Build history of the part. All positions in model axes, mm. A direction names the side the tool comes from. Round coordinates to 2 decimals unless told otherwise and drop trailing zeros. Write each loop counter-clockwise with the first axis right and the second up, starting at its lowest first coordinate (ties: lowest second). Pieces come first, ordered by that corner, then holes. Notation, with made-up numbers: M 57.5,-31 L 108.5,-31 A25 cw 108.5,-12 Z; hole C 39.25,-27.75 d2. An arc over 180 degrees is marked long. Use a Markdown table: item, result.
from build123d import *

# Parameters (mm, degrees)
FLOOR_2_DEPTH        = 40
SIDE_START           = 37
SKETCH_2_W           = 197.5
SKETCH_2_H           = 35
SIDE_FRONT_DEPTH     = 3
SIDE_START_2         = -37
SKETCH_3_W           = 197.5
SKETCH_3_H           = 35
SIDE_REAR_DEPTH      = 3
INSIDE_BEND_FRONT_R  = 3
INSIDE_BEND_REAR_R   = 3
OUTSIDE_BEND_FRONT_R = 6
OUTSIDE_BEND_REAR_R  = 6
JOINT_START          = 40
SKETCH_4_W           = 45
SKETCH_4_H           = 21
JOINT_FRONT_DEPTH    = 3
JOINT_START_2        = -40
SKETCH_5_W           = 45
SKETCH_5_H           = 21
JOINT_REAR_DEPTH     = 3
SKETCH_6_R           = 2.5
FIXING_HOLES_DEPTH   = 43


with BuildPart() as part:
    # 草图1 → Floor 2 (new, symmetric)
    with BuildSketch(Plane.XY):
        Polygon((-103.110079617, 0), (247.5, 0), (247.5, 3), (-103.962954093, 3), align=None)
    extrude(amount=FLOOR_2_DEPTH, both=True)

    # 草图2 → Side Front (add)
    with BuildSketch(Plane.XY.offset(SIDE_START)):
        with Locations((148.75, 20.5)):
            Rectangle(SKETCH_2_W, SKETCH_2_H)
    extrude(amount=SIDE_FRONT_DEPTH)

    # 草图3 → Side Rear (add)
    with BuildSketch(Plane.XY.offset(SIDE_START_2)):
        with Locations((148.75, 20.5)):
            Rectangle(SKETCH_3_W, SKETCH_3_H)
    extrude(amount=-SIDE_REAR_DEPTH)

    # Inside Bend Front
    inside_bend_front_edges = [part.edges().sort_by_distance(p)[0] for p in [
        (148.75, 3, 37),
    ]]
    fillet(inside_bend_front_edges, radius=INSIDE_BEND_FRONT_R)

    # Inside Bend Rear
    inside_bend_rear_edges = [part.edges().sort_by_distance(p)[0] for p in [
        (148.75, 3, -37),
    ]]
    fillet(inside_bend_rear_edges, radius=INSIDE_BEND_REAR_R)

    # Outside Bend Front
    outside_bend_front_edges = [part.edges().sort_by_distance(p)[0] for p in [
        (72.194960192, 0, 40),
    ]]
    fillet(outside_bend_front_edges, radius=OUTSIDE_BEND_FRONT_R)

    # Outside Bend Rear
    outside_bend_rear_edges = [part.edges().sort_by_distance(p)[0] for p in [
        (72.194960192, 0, -40),
    ]]
    fillet(outside_bend_rear_edges, radius=OUTSIDE_BEND_REAR_R)

    # 草图4 → Joint Front (add)
    with BuildSketch(Plane.XY.offset(JOINT_START)):
        with Locations((52.5, 20.5)):
            Rectangle(SKETCH_4_W, SKETCH_4_H)
    extrude(amount=JOINT_FRONT_DEPTH)

    # 草图5 → Joint Rear (add)
    with BuildSketch(Plane.XY.offset(JOINT_START_2)):
        with Locations((52.5, 20.5)):
            Rectangle(SKETCH_5_W, SKETCH_5_H)
    extrude(amount=-JOINT_REAR_DEPTH)

    # 草图6 → Fixing Holes (cut, symmetric)
    with BuildSketch(Plane.XY):
        with Locations((40, 20)):
            Circle(SKETCH_6_R)
        with Locations((65, 20)):
            Circle(SKETCH_6_R)
    extrude(amount=FIXING_HOLES_DEPTH, both=True, mode=Mode.SUBTRACT)


solid = part.part
Q1. Cut at C-C on x = 11.5. Give the cut face in (y, z).
Response values:
| item | result |
|---|---|
| outline | M 0,-34 A6 ccw 3,-39.2 L 3,39.2 A6 ccw 0,34 Z |
Q2. Cut at B-B on z = 15. Give the cut face in (x, y).
Response values:
| item | result |
|---|---|
| outline | M -103.96,3 L -103.11,0 L 247.5,0 L 247.5,3 Z |
Q3. Drop flat-ended pins along their axis: P1, Ø0.9, axis at y = 16.5, z = 42, coming from the +X side; P2, Ø6.5, axis at y = 22, z = 36, coming from the -X side; P3, Ø16, axis at x = 144, y = 27.5, coming from the +Z side; P4, Ø3, axis at x = 65, y = 20, coming from the -Z side. Give the stop position or say it passes through.
Response values:
| item | result |
|---|---|
| P1 | stops at x = 75 |
| P2 | stops at x = 50 |
| P3 | stops at z = 40 |
| P4 | passes through |
Q4. Which spindle directions (+Z, -Z, +X, -X, +Y, -Y) get a long thin tool onto all of the face, cutting with end or side? Do faces 4 (the flat face through (147, 22, -37)), 5 (the flat face through (40, 23, 40)), 6 (the flat face through (50, 20, 38)). Say none if no direction does.
Response values:
| item | result |
|---|---|
| face 4 | +X, -X, +Y |
| face 5 | -X, +Y, -Y |
| face 6 | -X, +Y |
Q5. Drill centre lines: L1, parallel to Z at x = 65, y = 23.5; L2, parallel to Y at x = 65, z = -40.95; L3, parallel to Y at x = 170, z = -9.5. Where is each one in solid material? Low to high.
Response values:
| item | result |
|---|---|
| L1 | z = -43 to -37, 37 to 43 |
| L2 | y = 10 to 17.5, 22.5 to 31 |
| L3 | y = 0 to 3 |
Q6. Two-plate mould, pull along Z, no slides. Class faces 1 (the flat face through (40, 23, -40)), 2 (the flat face through (52, 21, 43)), 3 (the flat face through (70, 0, 0)): +Z half, -Z half, draft (parallel to the pull), parting line (faces both ways), or undercut.
Response values:
| item | result |
|---|---|
| face 1 | undercut |
| face 2 | +Z half |
| face 3 | draft |
Q7. Cut at A-A on x = 174. Give the cut face in (y, z).
Response values:
| item | result |
|---|---|
| outline | M 0,-34 A6 ccw 6,-40 L 38,-40 L 38,-37 L 6,-37 A3 cw 3,-34 L 3,34 A3 cw 6,37 L 38,37 L 38,40 L 6,40 A6 ccw 0,34 Z |
